```python
from build123d import *

# Parameters (mm, degrees)
CUT_EXTRUDE1_START = -2.5
CUT_EXTRUDE1_DEPTH = 2.5


with BuildPart() as part:
    # Sketch2 → Revolve1 (revolve)
    with BuildSketch(Plane(origin=(0, 0, 0), x_dir=(0, 0, -1), z_dir=(1, 0, 0))):
        with BuildLine():
            Line((-20, 0), (-20, 3.967639565))
            ThreePointArc((-20, 3.967639565), (-19.994053088, 3.997536709), (-19.977117717, 4.022882283))
            Line((-19.977117717, 4.022882283), (-19.772882283, 4.227117717))
            ThreePointArc((-19.772882283, 4.227117717), (-19.747536709, 4.244053088), (-19.717639565, 4.25))
            Line((-19.717639565, 4.25), (-16.094860435, 4.25))
            ThreePointArc((-16.094860435, 4.25), (-16.064963291, 4.244053088), (-16.039617717, 4.227117717))
            Line((-16.039617717, 4.227117717), (-15.960382283, 4.147882283))
            ThreePointArc((-15.960382283, 4.147882283), (-15.935036709, 4.130946912), (-15.905139565, 4.125))
            Line((-15.905139565, 4.125), (-15.10625, 4.125))
            ThreePointArc((-15.10625, 4.125), (-15.031119904, 4.093880096), (-15, 4.01875))
            Line((-15, 4.01875), (-15, 2.75))
            ThreePointArc((-15, 2.75), (-14.926776695, 2.573223305), (-14.75, 2.5))
            Line((-14.75, 2.5), (19.480384758, 2.5))
            Line((19.480384758, 2.5), (20, 1.980384758))
            Line((20, 1.980384758), (20, 0))
            Line((20, 0), (-20, 0))
        make_face()
    revolve(axis=Axis((0, 0, -20), (0, 0, 1)))

    # Sketch3 → Cut-Extrude1 (cut)
    with BuildSketch(Plane.XY.offset(20).offset(CUT_EXTRUDE1_START)):
        Polygon((2, -1.154700538), (2, 1.154700538), (0, 2.309401077), (-2, 1.154700538), (-2, -1.154700538), (0, -2.309401077), align=None)
    extrude(amount=CUT_EXTRUDE1_DEPTH, mode=Mode.SUBTRACT)

    # Cut-Extrude2 cone 1 section (through the dimple's axis) → Cut-Extrude2 (revolve, cut)
    with BuildSketch(Plane(origin=(0, 0, 20), x_dir=(0, -1, 0), z_dir=(1, 0, 0))):
        Polygon((0, 0), (2.482606158, 0), (0, 2.482606158), align=None)
    revolve(axis=Axis((0, 0, 20), (0, 0, -1)), mode=Mode.SUBTRACT)


solid = part.part
```
Geometry check sheet. Reference: the model listing, model coordinates, mm. A direction names the side the tool comes from. Coordinates: 2 decimals unless noted, no trailing zeros. Write each loop counter-clockwise with the first axis right and the second up, starting at its lowest first coordinate (ties: lowest second). Pieces come first, ordered by that corner, then holes. Notation, with made-up numbers: M 72.25,59 L 131.25,59 A27 cw 131.25,80 Z; hole C 66.5,-28.75 d5. An arc over 180 degrees is marked long. Use one line per item in the form item = value. Start each with the question number.
1) Set-up check for faces 4 (the flat face through (0, 0, 17.5)), 5 (the flat face through (-2, -2, 20)), 6 (the flat face through (3, 1, 15)): record each of +Z, -Z, +X, -X, +Y, -Y from which the full face is reachable in a straight line by a thin tool's end or side.
2) Go/stop test with flat-tipped pins: pin 1 Ø2 at (x, y) = (1.5, 3) entering from -Z; pin 2 Ø1 at (x, y) = (-2, -2.5) entering from -Z; pin 3 Ø3 at (x, z) = (-3, 2) entering from +Y. Record where each tip stops, or that it passes through.
3) Section check B-B on z = -18. Enter the section's corners in (x, y).
4) Release check for a two-part mould opening along X. For faces 1 (the flat face through (0.99, -1.74, 18.65)), 2 (the cylindrical face through (-3.584, 2.285, 17.881)), 3 (the flat face through (0, 0, -20)) record: pulls with the +X half, pulls with the -X half, needs draft (parallel to the pull), parting line crosses it, or undercut.
5) Thickness scan on probe 1 along Z at (x, y) = (1, -3); probe 2 along X at (y, z) = (0, 1.5); probe 3 along Z at (x, y) = (1.25, -1.25). Record the ranges inside material, lowest first. Write a range as from..to.
Responses:
q1.face_4 = +Z
q1.face_5 = +Z, +X, -X, +Y, -Y
q1.face_6 = -Z
q2.pin_1 = -19.63
q2.pin_2 = 15
q2.pin_3 = 2
q3.outline = C 0,0 d5
q4.face_1 = undercut
q4.face_2 = parting line crosses it
q4.face_3 = needs draft
q5.probe_1 = 15..20
q5.probe_2 = -2.5..2.5
q5.probe_3 = -20..17.5
